For this review, take the finished solid that the model builds, in its own axes (mm). Face numbers are marked on the shaded views. A direction names the side the tool comes from. Give positions to 0.01 mm unless a question says otherwise; leave off trailing zeros. Loops run counter-clockwise (first coordinate to the right, second up) from the corner with the lowest first, then second, coordinate; pieces in that order, holes last.
```python
from build123d import *

# Parameters (mm, degrees)
BOSS_EXTRU_5_DEPTH       = 50
ESQUISSE5_R              = 2.15
ESQUISSE5_W              = 20
ESQUISSE5_H              = 31.8
ENL_V_MAT_EXTRU_1_DEPTH  = 10
BOSS_EXTRU_6_DEPTH       = 5
ESQUISSE11_R             = 2.5
ENL_V_MAT_EXTRU_9_DEPTH  = 5
CONG_1_R                 = 10
ENL_V_MAT_EXTRU_12_DEPTH = 12
ESQUISSE12_W             = 31
ESQUISSE12_H             = 23.2
ENL_V_MAT_EXTRU_13_DEPTH = 10
CONG_2_R                 = 1
ESQUISSE9_W              = 62
ESQUISSE9_H              = 34.999999956
ENL_V_MAT_EXTRU_14_DEPTH = 110.66312051
CONG_3_R                 = 5
CONG_4_R                 = 2
ESQUISSE13_R             = 1.5
ENL_V_MAT_EXTRU_15_DEPTH = 116.004347813
TROU_TARAUD_M31_D        = 2.5
TROU_TARAUD_M31_DEPTH    = 12.5
TROU_TARAUD_M31_TIP      = 0.751075774
ESQUISSE3D2_R            = 1.75
ENL_V_MAT_EXTRU_16_DEPTH = 8
ENL_V_MAT_EXTRU_17_DEPTH = 10


with BuildPart() as part:
    # Esquisse1 → Boss.-Extru.5 (new, symmetric)
    with BuildSketch(Plane(origin=(0, 0, 0), x_dir=(1, 0, 0), z_dir=(0, 1, 0))):
        Polygon((0, 31), (-40.496913463, 31), (-80, 31), (-80, -31), (-40.496913463, -31), (0, -31), (0, -26), (-40.496913463, -26), (-70, -26), (-70, 26), (-40.496913463, 26), (0, 26), align=None)
    extrude(amount=BOSS_EXTRU_5_DEPTH, both=True)

    # Esquisse5 → Enlèv. mat.-Extru.1 (cut)
    with BuildSketch(Plane(origin=(-70, 0, 0), x_dir=(0, 0, -1), z_dir=(1, 0, 0))):
        with BuildLine():
            Line((-10, -2), (10, -2))
            Line((10, -2), (10, 5.500000044))
            ThreePointArc((10, 5.500000044), (8.681980515, 8.68198056), (5.5, 10.000000044))
            Line((5.5, 10.000000044), (-5.499999911, 10.000000044))
            ThreePointArc((-5.499999911, 10.000000044), (-8.681980489, 8.681980534), (-10, 5.499999956))
            Line((-10, 5.499999956), (-10, -2))
        make_face()
        Circle(ESQUISSE5_R, mode=Mode.SUBTRACT)
        Circle(ESQUISSE5_R)
        with Locations((0, -17.9)):
            Rectangle(ESQUISSE5_W, ESQUISSE5_H)
        with BuildLine():
            ThreePointArc((2.15, 0), (-1.209582286, 1.77747312), (-0.788986692, -2))
            Line((-0.788986692, -2), (0.788986692, -2))
            ThreePointArc((0.788986692, -2), (1.77747312, -1.209582286), (2.15, 0))
        make_face()
        with BuildLine():
            Line((0.788986692, -2), (-0.788986692, -2))
            ThreePointArc((-0.788986692, -2), (0, -2.15), (0.788986692, -2))
        make_face()
    extrude(amount=-ENL_V_MAT_EXTRU_1_DEPTH, mode=Mode.SUBTRACT)

    # Esquisse8 → Boss.-Extru.6 (add)
    with BuildSketch(Plane(origin=(0, -50, 0), x_dir=(1, 0, 0), z_dir=(0, 1, 0))):
        with BuildLine():
            Line((0, -50.999999907), (0, 50.999999907))
            ThreePointArc((0, 50.999999907), (-22.584882388, 45.728136811), (-40.5, 31))
            Line((-40.5, 31), (-80, 31))
            Line((-80, 31), (-80, -31))
            Line((-80, -31), (-40.5, -31))
            ThreePointArc((-40.5, -31), (-22.584882388, -45.728136811), (0, -50.999999907))
        make_face()
    extrude(amount=-BOSS_EXTRU_6_DEPTH)

    # Esquisse11 → Enlèv. mat.-Extru.9 (cut)
    with BuildSketch(Plane(origin=(-70, 0, 0), x_dir=(0, 0, -1), z_dir=(1, 0, 0))):
        with Locations((-19.6, -22.213953616)):
            Circle(ESQUISSE11_R)
        with Locations((19.6, -22.213953616)):
            Circle(ESQUISSE11_R)
    extrude(amount=-ENL_V_MAT_EXTRU_9_DEPTH, mode=Mode.SUBTRACT)

    # Congé1
    cong_1_edges = [part.edges().sort_by_distance(p)[0] for p in [
        (-80, -2.5, 31),
        (-80, -2.5, -31),
    ]]
    fillet(cong_1_edges, radius=CONG_1_R)

    # Esquisse10 → Enlèv. mat.-Extru.12 (cut)
    with BuildSketch(Plane(origin=(0, 0, 0), x_dir=(0, 0, -1), z_dir=(1, 0, 0))):
        with BuildLine():
            Line((85.263165158, 65.69401727), (136.28713183, 33.486696785))
            ThreePointArc((136.28713183, 33.486696785), (0, -37), (-136.28713183, 33.486696785))
            Line((-136.28713183, 33.486696785), (-85.263165158, 65.69401727))
            ThreePointArc((-85.263165158, 65.69401727), (0, 23.205492896), (85.263165158, 65.69401727))
        make_face()
    extrude(amount=-ENL_V_MAT_EXTRU_12_DEPTH, mode=Mode.SUBTRACT)

    # Esquisse12 → Enlèv. mat.-Extru.13 (cut)
    with BuildSketch(Plane(origin=(0, -55, 0), x_dir=(-1, 0, 0), z_dir=(0, -1, 0))):
        with Locations((15.5, 0)):
            Rectangle(ESQUISSE12_W, ESQUISSE12_H)
    extrude(amount=-ENL_V_MAT_EXTRU_13_DEPTH, mode=Mode.SUBTRACT)

    # Congé2
    cong_2_edges = [part.edges().sort_by_distance(p)[0] for p in [
        (-15.5, -50, -11.6),
        (-31, -50, 0),
        (-15.5, -50, 11.6),
    ]]
    fillet(cong_2_edges, radius=CONG_2_R)

    # Esquisse9 → Enlèv. mat.-Extru.14 (cut, through all)
    with BuildSketch(Plane(origin=(0, 0, 0), x_dir=(0, 0, -1), z_dir=(1, 0, 0))):
        with Locations((0, 32.500000022)):
            Rectangle(ESQUISSE9_W, ESQUISSE9_H)
    extrude(amount=-ENL_V_MAT_EXTRU_14_DEPTH, mode=Mode.SUBTRACT)

    # Congé3
    cong_3_edges = [part.edges().sort_by_distance(p)[0] for p in [
        (-55.25, -55, 31),
        (-77.071067812, -55, 28.071067812),
        (-80, -55, 0),
        (-77.071067812, -55, -28.071067812),
        (-55.25, -55, -31),
    ]]
    fillet(cong_3_edges, radius=CONG_3_R)

    # Congé4
    cong_4_edges = [part.edges().sort_by_distance(p)[0] for p in [
        (-12, 15.000000044, 28.5),
        (-77.071067812, 15.000000044, 28.071067812),
        (-77.071067812, 15.000000044, -28.071067812),
        (-12, 15.000000044, -28.5),
        (-41, 15.000000044, 26),
        (-70, 15.000000044, 0),
        (-41, 15.000000044, 31),
        (-80, 15.000000044, 0),
        (-41, 15.000000044, -31),
        (-41, 15.000000044, -26),
    ]]
    fillet(cong_4_edges, radius=CONG_4_R)

    # Esquisse13 → Enlèv. mat.-Extru.15 (cut, through all)
    with BuildSketch(Plane(origin=(0, -50, 0), x_dir=(1, 0, 0), z_dir=(0, 1, 0))):
        with Locations(Location((-21, 40.999999953, 0), (0, 0, 270))):
            Circle(ESQUISSE13_R)
        with Locations(Location((-6, 40.999999953, 0), (0, 0, 270))):
            Circle(ESQUISSE13_R)
        with Locations(Location((-6, -40.999999953, 0), (0, 0, 90))):
            Circle(ESQUISSE13_R)
        with Locations(Location((-21, -40.999999953, 0), (0, 0, 90))):
            Circle(ESQUISSE13_R)
    extrude(amount=-ENL_V_MAT_EXTRU_15_DEPTH, mode=Mode.SUBTRACT)

    # Trou taraudé M31
    with Locations(Plane(origin=(-70, -6.5, 13.5), x_dir=(0, 0, 1), z_dir=(1, 0, 0))):
        with Locations((0, 0), (-27, 0), (-27, 8), (0, 8), (0, 16), (-27, 16), (-27, 24), (0, 24)):
            Hole(TROU_TARAUD_M31_D / 2, depth=TROU_TARAUD_M31_DEPTH)
            with Locations((0, 0, -(TROU_TARAUD_M31_DEPTH + TROU_TARAUD_M31_TIP / 2))):  # 118° drill point
                Cone(0, TROU_TARAUD_M31_D / 2, TROU_TARAUD_M31_TIP, mode=Mode.SUBTRACT)

    # Esquisse3D2 → Enlèv. mat.-Extru.16 (cut)
    with BuildSketch(Plane(origin=(-80, -6.5, 13.5), x_dir=(0, -0.6643638388299197, -0.7474093186836598), z_dir=(-1, 0, 0))):
        with Locations(Location((0, 0, 0), (0, 0, 318.366460663))):
            Circle(ESQUISSE3D2_R)
        with Locations(Location((5.314910711, 5.979274549, 0), (0, 0, 318.366460663))):
            Circle(ESQUISSE3D2_R)
        with Locations(Location((10.629821421, 11.958549099, 0), (0, 0, 318.366460663))):
            Circle(ESQUISSE3D2_R)
        with Locations(Location((20.180051604, -17.937823648, 0), (0, 0, 318.366460663))):
            Circle(ESQUISSE3D2_R)
        with Locations(Location((25.494962315, -11.958549099, 0), (0, 0, 318.366460663))):
            Circle(ESQUISSE3D2_R)
        with Locations(Location((30.809873026, -5.979274549, 0), (0, 0, 318.366460663))):
            Circle(ESQUISSE3D2_R)
        with Locations(Location((36.124783736, 0, 0), (0, 0, 318.366460663))):
            Circle(ESQUISSE3D2_R)
        with Locations(Location((15.944732132, 17.937823648, 0), (0, 0, 318.366460663))):
            Circle(ESQUISSE3D2_R)
    extrude(amount=-ENL_V_MAT_EXTRU_16_DEPTH, mode=Mode.SUBTRACT)

    # Esquisse3D3 → Enlèv. mat.-Extru.17 (cut)
    with BuildSketch(Plane(origin=(-80, -44, 6), x_dir=(0, -0.4472135954999578, -0.894427190999916), z_dir=(1, 0, 0))):
        Polygon((0, 0), (10.733126292, 5.366563146), (13.416407865, 0), (2.683281573, -5.366563146), align=None)
    extrude(amount=ENL_V_MAT_EXTRU_17_DEPTH, mode=Mode.SUBTRACT)


solid = part.part
```
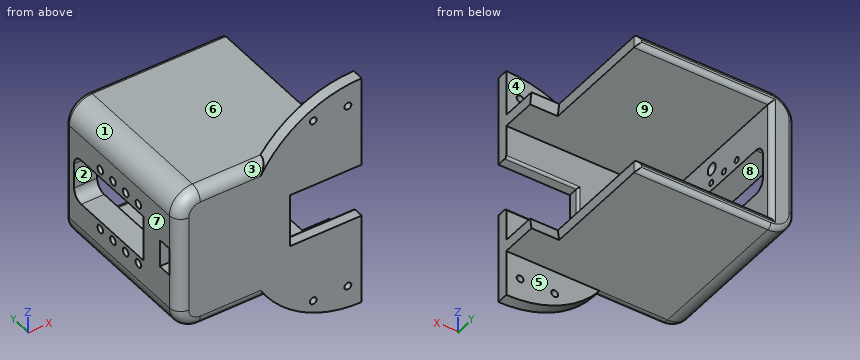
Q1. Consider section D-D on z = 19.6. Give the boundary of the cut face in (x, y).
Answers:
outline: (-80, -50) arc R5 ccw to (-75, -55) - (0, -55) - (0, -50) - (-70, -50) - (-70, -24.71) - (-75, -24.71) - (-75, -19.71) - (-70, -19.71) - (-70, 13) arc R2 ccw to (-72, 15) - (-78, 15) arc R2 ccw to (-80, 13) - close
Q2. Consider section A-A on y = -26. Give the boundary of the cut face in (x, z), plus the area to 3 significant figures.
Answers:
outline: (-80, -21) arc R10 ccw to (-70, -31) - (-12, -31) - (-12, -26) - (-70, -26) - (-70, -10) - (-80, -10) - close; (-80, 10) - (-70, 10) - (-70, 26) - (-12, 26) - (-12, 31) - (-70, 31) arc R10 ccw to (-80, 21) - close
area: 957 mm2
Q3. Mouldability with a two-part tool opening along Y and no side actions: class the marked faces 1, 2, 3 and 4 as +Y half, -Y half, draft (parallel to the pull), parting line (faces both ways), or undercut.
Answers:
face 1: draft
face 2: undercut
face 3: -Y half
face 4: +Y half
Q4. Consider section B-B on z = 1. Give the boundary of the cut face in (x, y), plus the area to 3 significant figures.
Answers:
outline: (-80, -50) arc R5 ccw to (-75, -55) - (-31, -55) - (-31, -51) arc R1 ccw to (-32, -50) - close; (-80, -44) - (-70, -44) - (-70, -33.8) - (-80, -33.8) - close; (-80, 10) - (-70, 10) - (-70, 13) arc R2 ccw to (-72, 15) - (-78, 15) arc R2 ccw to (-80, 13) - close
area: 390 mm2
Q5. For pin 1 Ø8 at (x, z) = (-31, 8.5) entering from +Y; pin 2 Ø1.8 at (x, z) = (-6, 41) entering from -Y (3 decimals); pin 3 Ø3 at (y, z) = (-30.5, 13.5) entering from -X; pin 4 Ø3 at (x, y) = (-17.5, 0.5) entering from -Z, all flat-tipped, find the tip position at first contact; note any pin that passes through.
Answers:
pin 1: stops at y = -50
pin 2: passes through
pin 3: stops at x = -72
pin 4: stops at z = -31
Q6. For probe 1 along Z at (x, y) = (-70.75, -14.5); probe 2 along Y at (x, z) = (-72.2, 19.6); probe 3 along Z at (x, y) = (-42, 0), list the stretches that pass through material, from the lowest coordinate up.
Answers:
probe 1: z = -30.97 to -14.75, -12.25 to -10, 10 to 12.25, 14.75 to 30.97
probe 2: y = -55 to -24.71, -19.71 to 15
probe 3: z = -31 to -26, 26 to 31
Q7. Consider section C-C on x = -21. Count the separate pieces of the cut face and the enclosed holes in it, plus the area to 3 significant figures.
Answers:
separate pieces: 4
enclosed holes: 0
area: 965 mm2
Q8. Machinability: for the marked faces 5, 6, 7, 8 and 9, which of the approach directions +Z, -Z, +X, -X, +Y, -Y give a long, thin tool a straight path to every point of the face, cutting with its end or side? Answer none if there is none.
Answers:
face 5: -Z, +X, -X, +Y
face 6: +Z, +X, -X, +Y
face 7: +Z, -Z, -X, +Y, -Y
face 8: +X, -X
face 9: +X, +Y
